```python
from build123d import *

# Parameters (mm, degrees)
SKETCH_1_R          = 3.5
EXTRUDE_1_DEPTH     = 15
CUT_EXTRUDE_1_DEPTH = 3.2
CUT_EXTRUDE_2_DEPTH = 3
CUT_EXTRUDE_3_DEPTH = 3
SKETCH_5_R          = 2.5
CUT_EXTRUDE_4_DEPTH = 15
SKETCH_6_R          = 2
CUT_EXTRUDE_5_DEPTH = 15


with BuildPart() as part:
    # Эскиз1 → Вытянуть1 (new body)
    with BuildSketch(Plane.XY):
        with BuildLine():
            Line((-33.737889323, 6), (0, 8))
            ThreePointArc((0, 8), (8, 0), (0, -8))
            Line((0, -8), (-33.737889323, -6))
            ThreePointArc((-33.737889323, -6), (-39.737889323, 0), (-33.737889323, 6))
        make_face()
        Circle(SKETCH_1_R, mode=Mode.SUBTRACT)
    extrude(amount=EXTRUDE_1_DEPTH)

    # Эскиз2 → Вырез-Вытянуть1 (cut)
    with BuildSketch(Plane.XY.offset(9.1)):
        with BuildLine():
            Line((-21.470788926, 6.727200228), (-0.649375953, 7.973600872))
            Line((-0.649375953, 7.973600872), (-0.649375953, 12.464774984))
            Line((-0.649375953, 12.464774984), (11.53167748, 12.464774984))
            Line((11.53167748, 12.464774984), (11.53167748, -11.583586667))
            Line((11.53167748, -11.583586667), (-0.649375953, -11.583586667))
            Line((-0.649375953, -11.583586667), (-0.649375953, -7.973600872))
            Line((-0.649375953, -7.973600872), (-21.470788926, -6.727200228))
            ThreePointArc((-21.470788926, -6.727200228), (-22.5, 0), (-21.470788926, 6.727200228))
        make_face()
    extrude(amount=-CUT_EXTRUDE_1_DEPTH, mode=Mode.SUBTRACT)

    # Эскиз3 → Вырез-Вытянуть2 (cut)
    with BuildSketch(Plane.XY.offset(15)):
        with BuildLine():
            Line((-58.585224431, 9.320685439), (-23.289981774, 9.320685439))
            ThreePointArc((-23.289981774, 9.320685439), (-24.945775434, 0.205603355), (-23.289981774, -8.909478729))
            Line((-23.289981774, -8.909478729), (-58.585224431, -8.909478729))
            Line((-58.585224431, -8.909478729), (-58.585224431, 9.320685439))
        make_face()
    extrude(amount=-CUT_EXTRUDE_2_DEPTH, mode=Mode.SUBTRACT)

    # Эскиз4 → Вырез-Вытянуть3 (cut)
    with BuildSketch(Plane(origin=(0, 0, 0), x_dir=(-1, 0, 0), z_dir=(0, 0, -1))):
        with BuildLine():
            Line((7.501860508, 8.168918957), (7.501860508, 9.225490058))
            Line((7.501860508, 9.225490058), (56.423561983, 9.225490058))
            Line((56.423561983, 9.225490058), (56.423561983, -10.745771297))
            Line((56.423561983, -10.745771297), (16.608517708, -10.745771297))
            Line((16.608517708, -10.745771297), (16.608517708, -7.871583169))
            add(Edge.make_bspline(
                [(7.501860508, 8.168918957), (26.545638359, 4.198485706), (16.608517708, -7.871583169)],
                knots=[0, 0, 0, 1, 1, 1], degree=2))
        make_face()
    extrude(amount=-CUT_EXTRUDE_3_DEPTH, mode=Mode.SUBTRACT)

    # Эскиз5 → Вырез-Вытянуть4 (cut)
    with BuildSketch(Plane.XY.offset(12)):
        with Locations((-33.737889323, 0)):
            Circle(SKETCH_5_R)
    extrude(amount=-CUT_EXTRUDE_4_DEPTH, mode=Mode.SUBTRACT)

    # Эскиз6 → Вырез-Вытянуть5 (cut)
    with BuildSketch(Plane.XY.offset(15)):
        with Locations((-17.165585922, 0)):
            Circle(SKETCH_6_R)
    extrude(amount=-CUT_EXTRUDE_5_DEPTH, mode=Mode.SUBTRACT)


solid = part.part
```
Read the model definition and answer for the solid it produces. Units are mm, in the model's axes. A direction names the side the tool comes from. Coordinates: 2 decimals unless noted, no trailing zeros. Write each loop counter-clockwise with the first axis right and the second up, starting at its lowest first coordinate (ties: lowest second). Pieces come first, ordered by that corner, then holes. Notation, with made-up numbers: (51.25, 74) -> (85.25, 74) arc R26 ccw to (85.25, 88) -> close; hole circle Ø9 at (-13.5, 21.25). An arc over 180 degrees is marked (long way). Return JSON: item names as keys, results as strings.
1. A cutting plane is placed at B-B (x = 5.5). Determine the outline of the cut face in (y, z), and give its area (3 significant figures).
Found:
{"outline": "(-5.81, 0) -> (5.81, 0) -> (5.81, 5.9) -> (-5.81, 5.9) -> close; (-5.81, 9.1) -> (5.81, 9.1) -> (5.81, 15) -> (-5.81, 15) -> close", "area": "137 mm2"}
2. Determine the mould class of faces 3 (the face through (-24.945, 0.083, 13.521)), 4 (the face through (-7, 0, 5.9)), 5 (the face through (3.233, -1.341, 12.009)) for opening direction X: pulls with the +X half, pulls with the -X half, needs draft (parallel to the pull), parting line crosses it, or undercut.
Found:
{"face 3": "pulls with the -X half", "face 4": "needs draft", "face 5": "undercut"}
3. Each of these flat-tipped pins is pushed along its axis until it touches: P1, Ø1, axis at y = 5, z = 6.5, coming from the -X side; P2, Ø6, axis at y = 1, z = 3.5, coming from the -X side; P3, Ø8, axis at x = -30, y = -4.5, coming from the -Z side; P4, Ø2, axis at y = 1, z = 7.5, coming from the +X side. Where does it stop, or does it pass through?
Found:
{"P1": "x = -37.71", "P2": "x = -39.74", "P3": "z = 3", "P4": "x = -22.41"}
4. Find the intervals of material crossed by line 1 along Z through (x, y) = (-20.5, -5.5); line 2 along Z through (x, y) = (-11, -6.25); line 3 along Z through (x, y) = (-23.5, 3.25), in increasing order. Write a range as from..to.
Found:
{"line 1": "3..5.9, 9.1..15", "line 2": "0..5.9, 9.1..15", "line 3": "3..15"}
5. A tool of negligible diameter and unlimited length cuts with its end or side. For faces 1 (the face through (-22.5, -0.1, 7.5)), 2 (the face through (-19.164, 0.088, 12.091)), from which of +Z, -Z, +X, -X, +Y, -Y can it reach the whole face along a straight path? Write none if from no direction.
Found:
{"face 1": "+X", "face 2": "+Z, -Z"}
6. A cutting plane is placed at C-C (y = 0). Give the number of separate pieces and of enclosed holes in the cut face, and give its area (3 significant figures).
Found:
{"separate pieces": "6", "enclosed holes": "0", "area": "340 mm2"}
7. A cutting plane is placed at A-A (z = 4). Determine the outline of the cut face in (x, y).
Found:
{"outline": "(-33.74, -6) -> (0, -8) arc R8 ccw to (0, 8) -> (-33.74, 6) arc R6 ccw to start; hole circle Ø5 at (-33.74, 0); hole circle Ø4 at (-17.17, 0); hole circle Ø7 at (0, 0)"}
